from build123d import *

# Parameters (mm, degrees)
PROFILE_LASER_PROFILE_3P5_R   = 2.2
PROFILE_LASER_PROFILE_3P5_R_2 = 0.9
PROFILE_LASER_PROFILE_3P5_W   = 3.5
PROFILE_LASER_PROFILE_3P5_H   = 3
PROFILE_LASER_PROFILE_3P5_W_2 = 6
PROFILE_LASER_PROFILE_3P5_H_2 = 3.5
LASER_PROFILE_3P5_DEPTH       = 3.5


with BuildPart() as part:
    # Profile_Laser_profile_3p5 → Laser_profile_3p5 (new body)
    with BuildSketch(Plane.XY):
        Polygon((0, 30.427227289), (8, 18), (4, 18), (12, 7), (10, 7), (14, -7), (10, -7), (14, -20), (10, -20), (14, -33), (4, -33), (4, -49.572772711), (-4, -49.572772711), (-4, -33), (-14, -33), (-10, -20), (-14, -20), (-10, -7), (-14, -7), (-10, 7), (-12, 7), (-4, 18), (-8, 18), align=None)
        Circle(PROFILE_LASER_PROFILE_3P5_R, mode=Mode.SUBTRACT)
        with Locations((0, -4.5)):
            Circle(PROFILE_LASER_PROFILE_3P5_R_2, mode=Mode.SUBTRACT)
        with Locations((0, 4.5)):
            Circle(PROFILE_LASER_PROFILE_3P5_R_2, mode=Mode.SUBTRACT)
        with Locations((-7, 3.5)):
            Rectangle(PROFILE_LASER_PROFILE_3P5_W, PROFILE_LASER_PROFILE_3P5_H, mode=Mode.SUBTRACT)
        with Locations((-7, -2.5)):
            Rectangle(PROFILE_LASER_PROFILE_3P5_W, PROFILE_LASER_PROFILE_3P5_H, mode=Mode.SUBTRACT)
        with Locations((-7, -25.5)):
            Rectangle(PROFILE_LASER_PROFILE_3P5_W, PROFILE_LASER_PROFILE_3P5_H, mode=Mode.SUBTRACT)
        with Locations((7, 3.5)):
            Rectangle(PROFILE_LASER_PROFILE_3P5_W, PROFILE_LASER_PROFILE_3P5_H, mode=Mode.SUBTRACT)
        with Locations((7, -2.5)):
            Rectangle(PROFILE_LASER_PROFILE_3P5_W, PROFILE_LASER_PROFILE_3P5_H, mode=Mode.SUBTRACT)
        with Locations((7, -25.5)):
            Rectangle(PROFILE_LASER_PROFILE_3P5_W, PROFILE_LASER_PROFILE_3P5_H, mode=Mode.SUBTRACT)
        with Locations((0, -10.25)):
            Rectangle(PROFILE_LASER_PROFILE_3P5_W_2, PROFILE_LASER_PROFILE_3P5_H_2, mode=Mode.SUBTRACT)
    extrude(amount=LASER_PROFILE_3P5_DEPTH)


solid = part.part
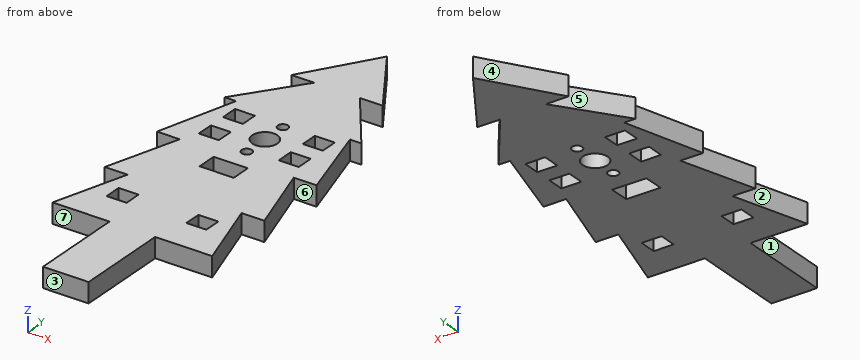
Source: CAD feature listing. Evaluate the final solid. Frame: model axes, mm. Face numbers are marked on the shaded views. A direction names the side the tool comes from. Round coordinates to 2 decimals unless told otherwise and drop trailing zeros. Loops run counter-clockwise (first coordinate to the right, second up) from the corner with the lowest first, then second, coordinate; pieces in that order, holes last.
Q1. First-contact query: P1, Ø1.5, axis at y = -2.5, z = 2, coming from the +X side; P2, Ø0.9, axis at y = -2, z = 2, coming from the +X side; P3, Ø1.8, axis at x = 6.5, z = 1.5, coming from the +Y side; P4, Ø12, axis at x = 3, y = -29, coming from the -Z side. Flat tips, straight axial feed; report the tip coordinate or a pass-through.
Q2. Section C-C, the plane y = -35. Return loops of the section in (x, z), plus the area to 3 significant figures.
Q3. Section D-D, the plane y = 13.5. Return loops of the section in (x, z).
Q4. Section B-B, the plane z = 2.25. State how many separate pieces and enclosed holes the cut face has, plus the area to 3 significant figures.
Q5. Mould query, pull axis Y, two halves, no side actions, for the marked faces 1, 2, 3 and 4. Classes: pulls with the +Y half, pulls with the -Y half, needs draft (parallel to the pull), parting line crosses it, or undercut.
Q6. Section A-A, the plane y = 0. Return loops of the section in (x, z), plus the area to 3 significant figures.
Q7. Ray query, line 1 (Y direction, x = 6, z = 3.35); line 2 (Y direction, x = 0.5, z = 0.5); line 3 (X direction, y = -44.5, z = 1.7). Return the intervals inside material, ascending.
Q8. Access query for the marked faces 5, 6 and 7. Directions: +Z, -Z, +X, -X, +Y, -Y. A direction counts if a zero-diameter tool reaches every point of the face in a straight line with its end or side. Return the directions, or none.
Solutions:
1. P1: stops at x = 12.93
1. P2: stops at x = 12.7
1. P3: stops at y = 21.73
1. P4: stops at z = 0
2. outline: (-4, 0) - (4, 0) - (4, 3.5) - (-4, 3.5) - close
2. area: 28.0 mm2
3. outline: (-7.27, 0) - (7.27, 0) - (7.27, 3.5) - (-7.27, 3.5) - close
4. separate pieces: 1
4. enclosed holes: 10
4. area: 1,260 mm2
5. face 1: needs draft
5. face 2: undercut
5. face 3: pulls with the -Y half
5. face 4: pulls with the +Y half
6. outline: (-12, 0) - (-2.2, 0) - (-2.2, 3.5) - (-12, 3.5) - close; (2.2, 0) - (12, 0) - (12, 3.5) - (2.2, 3.5) - close
6. area: 68.6 mm2
7. line 1: y = -33 to -27, -24 to -4, -1 to 2, 5 to 15.25, 18 to 21.11
7. line 2: y = -49.57 to -12, -8.5 to -5.25, -3.75 to -2.14, 2.14 to 3.75, 5.25 to 29.65
7. line 3: x = -4 to 4
8. face 5: +Z, -Z, -X
8. face 6: +Z, -Z, +X
8. face 7: +Z, -Z, -X, -Y
